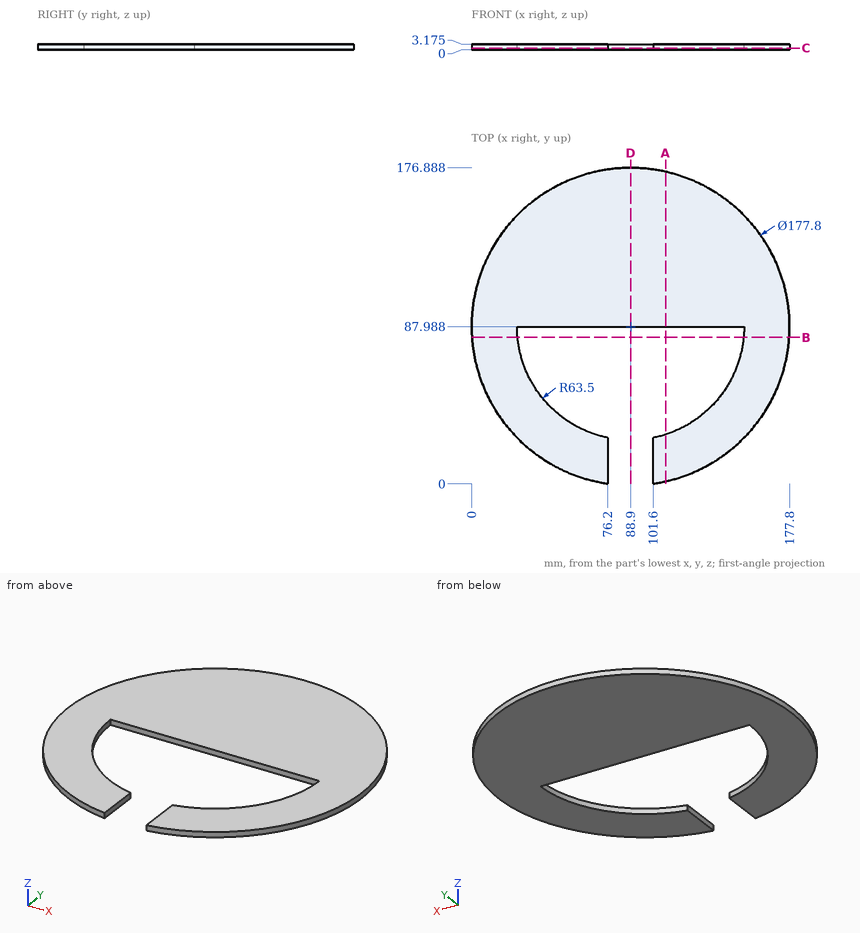
Input: dimensioned drawing with shaded views. Units: mm. Origin: part minimum x, y, z. Give positions to 0.01 mm unless a question says otherwise; leave off trailing zeros. Order: outer loops, then holes, each group sorted by start corner. A loop starts at its lowest first (then second) coordinate and runs counter-clockwise, first axis right, second up.
(1) Contact query for flat-ended pins moving along their axis: P1, Ø1.6, axis at y = 19, z = 1.5, coming from the -X side; P2, Ø1, axis at x = 29, z = 1, coming from the -Y side (1 decimal). Output: stop coordinate, or through.
(2) Section query C-C (z = 0.8). Return the cut outline in (x, y).
(3) Section query D-D (x = 88.9). Return the cut outline in (y, z) (1 decimal), plus the area to 3 significant figures.
(4) Section query A-A (x = 108.5). Return the cut outline in (y, z) (1 decimal), plus the area to 3 significant figures.
(5) Material intervals for line 1 along Y through (x, z) = (89.5, 0.6); line 2 along Y through (x, z) = (73.5, 2.7); line 3 along Y through (x, z) = (131, 0.2), sorted ascending.
(6) Section query B-B (y = 82). Return the cut outline in (x, z) (3 decimals).
Outcome:
1. P1: stops at x = 31.86
1. P2: stops at y = 21.8
2. outline: (25.4, 87.99) - (152.4, 87.99) arc R63.5 cw to (101.6, 25.77) - (101.6, 0) arc R88.9 ccw (long way) to (76.2, 0) - (76.2, 25.77) arc R63.5 cw to start
3. outline: (88, 0) - (176.9, 0) - (176.9, 3.2) - (88, 3.2) - close
3. area: 282 mm2
4. outline: (1.3, 0) - (27.6, 0) - (27.6, 3.2) - (1.3, 3.2) - close; (88, 0) - (174.7, 0) - (174.7, 3.2) - (88, 3.2) - close
4. area: 359 mm2
5. line 1: y = 87.99 to 176.89
5. line 2: y = 0.43 to 26.38, 87.99 to 175.54
5. line 3: y = 9.69 to 40.45, 87.99 to 166.29
6. outline: (0.202, 0) - (25.683, 0) - (25.683, 3.175) - (0.202, 3.175) - close; (152.117, 0) - (177.598, 0) - (177.598, 3.175) - (152.117, 3.175) - close
